from build123d import *

# Parameters (mm, degrees)
SKETCH2_W               = 15.875
SKETCH2_H               = 79.375
SKETCH2_R               = 1.7272
SKETCH2_W_2             = 25.4
SKETCH2_H_2             = 6.35
BOSS_EXTRUDE1_DEPTH     = 69.85
SKETCH3_W               = 19.05
SKETCH3_H               = 12.7
CUT_EXTRUDE1_DEPTH      = 127
SKETCH4_R               = 2.2950679
CUT_EXTRUDE2_DEPTH      = 127
CHAMFER1_SIZE           = 6.35
FILLET2_R               = 6.35
CUT_EXTRUDE3_DEPTH      = 6.35
CUT_EXTRUDE3_DEPTH_BACK = 6.35
SKETCH8_R               = 2.4
SKETCH10_W              = 9.525
SKETCH10_H              = 4.699
BOSS_EXTRUDE2_DEPTH     = 12.7
SKETCH12_R              = 0.8763
CUT_EXTRUDE4_DEPTH      = 132.769283049
CHAMFER2_SIZE           = 4.7752
CHAMFER2_SIZE_2         = 12.7
CHAMFER3_SIZE           = 4.70154
CHAMFER4_SIZE           = 6.35
CHAMFER4_SIZE_2         = 12.7
CUT_EXTRUDE5_DEPTH      = 0.254
CUT_EXTRUDE6_DEPTH      = 0.254


# Some blends are built 0.0001 mm under size
with BuildPart() as part:
    # Sketch2 → Boss-Extrude1 (new body)
    # profile 1 of 2: a face of its own
    with BuildSketch(Plane.ZY.offset(62.053242547)):
        with Locations((17.149745439, 79.910239505)):
            Rectangle(SKETCH2_W, SKETCH2_H)
        with Locations((17.149745439, 113.247739505)):
            Circle(SKETCH2_R, mode=Mode.SUBTRACT)
        with Locations((17.149745439, 71.972739505)):
            Circle(SKETCH2_R, mode=Mode.SUBTRACT)
    # profile 2 of 2: a face of its own
    with BuildSketch(Plane.ZY.offset(62.053242547)):
        with Locations((-3.487754561, 68.797739505)):
            Rectangle(SKETCH2_W_2, SKETCH2_H_2)
    extrude(amount=-BOSS_EXTRUDE1_DEPTH)

    # Sketch3 → Cut-Extrude1 (cut)
    with BuildSketch(Plane(origin=(0, 0, 9.212245439), x_dir=(-1, 0, 0), z_dir=(0, 0, -1))):
        with Locations((27.128242547, 52.922739505)):
            Rectangle(SKETCH3_W, SKETCH3_H)
    extrude(amount=-CUT_EXTRUDE1_DEPTH, mode=Mode.SUBTRACT)

    # Sketch4 → Cut-Extrude2 (cut)
    with BuildSketch(Plane(origin=(7.796757453, 0, 0), x_dir=(0, 0, -1), z_dir=(1, 0, 0))):
        with Locations(Location((-17.149745439, 52.922739505, 0), (0, 0, 180))):
            Circle(SKETCH4_R)
    extrude(amount=-CUT_EXTRUDE2_DEPTH, mode=Mode.SUBTRACT)

    # Chamfer1
    chamfer1_edges = [part.edges().sort_by_distance(p)[0] for p in [
        (-27.128242547, 59.272739505, 25.087245439),
        (-27.128242547, 46.572739505, 9.212245439),
    ]]
    chamfer(chamfer1_edges, length=CHAMFER1_SIZE - 0.0001)  # a hair under: the kernel refuses the full size

    # Fillet2
    fillet2_edges = [part.edges().sort_by_distance(p)[0] for p in [
        (-27.128242547, 59.272739505, 18.737345439),
        (-27.128242547, 46.572739505, 15.562145439),
    ]]
    fillet(fillet2_edges, radius=FILLET2_R)

    # Sketch8 → Cut-Extrude3 (cut, two sides: drawn at the far end of the back side and taken through both)
    # profile 1 of 5: a face of its own
    with BuildSketch(Plane(origin=(-27.128242547, 59.272739505, 33.482952844), x_dir=(0, 0, 1), z_dir=(-1, 0, 0)).offset(-CUT_EXTRUDE3_DEPTH_BACK)):
        with BuildLine():
            Line((-7.077924175, -7.789561181), (-20.085542155, 7.712314277))
            ThreePointArc((-20.085542155, 7.712314277), (-21.190808514, 7.041102183), (-22.339064084, 6.446418612))
            Line((-22.339064084, 6.446418612), (-9.023677061, -9.422241709))
            Line((-9.023677061, -9.422241709), (-7.077924175, -7.789561181))
        make_face()
    # profile 2 of 5: a face of its own
    with BuildSketch(Plane(origin=(-27.128242547, 59.272739505, 33.482952844), x_dir=(0, 0, 1), z_dir=(-1, 0, 0)).offset(-CUT_EXTRUDE3_DEPTH_BACK)):
        with BuildLine():
            Line((-20.085542155, 7.712314277), (-24.270707405, 12.7))
            Line((-24.270707405, 12.7), (-26.21646029, 11.067319471))
            Line((-26.21646029, 11.067319471), (-22.339064084, 6.446418612))
            ThreePointArc((-22.339064084, 6.446418612), (-21.190808514, 7.041102183), (-20.085542155, 7.712314277))
        make_face()
    # profile 3 of 5: a face of its own
    with BuildSketch(Plane(origin=(-27.128242547, 59.272739505, 33.482952844), x_dir=(0, 0, 1), z_dir=(-1, 0, 0)).offset(-CUT_EXTRUDE3_DEPTH_BACK)):
        Polygon((-26.21646029, 11.067319471), (-24.270707405, 12.7), (-27.58644192, 12.7), align=None)
    # profile 4 of 5: a face of its own
    with BuildSketch(Plane(origin=(-27.128242547, 59.272739505, 33.482952844), x_dir=(0, 0, 1), z_dir=(-1, 0, 0)).offset(-CUT_EXTRUDE3_DEPTH_BACK)):
        with BuildLine():
            ThreePointArc((-11.470707405, 23.65), (-13.762240918, 14.591506693), (-20.085542155, 7.712314277))
            Line((-20.085542155, 7.712314277), (-7.077924175, -7.789561181))
            Line((-7.077924175, -7.789561181), (9.239394359, 5.902294783))
            Line((9.239394359, 5.902294783), (-15.927560764, 35.895103965))
            ThreePointArc((-15.927560764, 35.895103965), (-12.619562979, 30.16548373), (-11.470707405, 23.65))
        make_face()
    # profile 5 of 5: a face of its own
    with BuildSketch(Plane(origin=(-27.128242547, 59.272739505, 33.482952844), x_dir=(0, 0, 1), z_dir=(-1, 0, 0)).offset(-CUT_EXTRUDE3_DEPTH_BACK)):
        with BuildLine():
            Line((-27.58644192, 12.7), (-24.270707405, 12.7))
            Line((-24.270707405, 12.7), (-20.085542155, 7.712314277))
            ThreePointArc((-20.085542155, 7.712314277), (-13.762240918, 14.591506693), (-11.470707405, 23.65))
            ThreePointArc((-11.470707405, 23.65), (-12.619562979, 30.16548373), (-15.927560764, 35.895103965))
            ThreePointArc((-15.927560764, 35.895103965), (-42.128931765, 38.754688915), (-46.109164673, 12.7))
            Line((-46.109164673, 12.7), (-27.58644192, 12.7))
        make_face()
        with Locations((-30.520707405, 23.65)):
            Circle(SKETCH8_R, mode=Mode.SUBTRACT)
    extrude(amount=CUT_EXTRUDE3_DEPTH + CUT_EXTRUDE3_DEPTH_BACK, mode=Mode.SUBTRACT)

    # Sketch10 → Boss-Extrude2 (add)
    with BuildSketch(Plane(origin=(0, 0, 9.212245439), x_dir=(-1, 0, 0), z_dir=(0, 0, -1))):
        with Locations((46.262342601, 74.322239505)):
            Rectangle(SKETCH10_W, SKETCH10_H)
        with Locations((46.262342601, 102.311439505)):
            Rectangle(SKETCH10_W, SKETCH10_H)
    extrude(amount=BOSS_EXTRUDE2_DEPTH)

    # Sketch12 → Cut-Extrude4 (cut, through all)
    with BuildSketch(Plane(origin=(-41.499842601, 0, 0), x_dir=(0, 0, -1), z_dir=(1, 0, 0))):
        with Locations((-2.862245439, 101.816839505)):
            Circle(SKETCH12_R)
        with Locations((-2.862245439, 74.816839505)):
            Circle(SKETCH12_R)
    extrude(amount=-CUT_EXTRUDE4_DEPTH, mode=Mode.SUBTRACT)

    # Chamfer2
    # the kernel refuses this chamfer: 12.7, 4.7752 mm, written as the material it adds along each edge
    with BuildSketch(Plane(origin=(-41.499842601, 104.660939505, 9.212245439), x_dir=(0, 0.9954252149618871, 0.09554392402492679), z_dir=(-1, 0, 0))) as chamfer2_piece_1:
        Polygon((CHAMFER2_SIZE * 0.995425214962, CHAMFER2_SIZE * 0.0955439240249), (-CHAMFER2_SIZE_2 * 0.0955439240249, CHAMFER2_SIZE_2 * 0.995425214962), (0, 0), align=None)
    extrude(amount=9.525)

    # Chamfer3
    # the kernel refuses this chamfer: 4.70154 mm, written as the material it adds along each edge
    with BuildSketch(Plane(origin=(-62.053242547, 71.972739505, 9.212245439), x_dir=(0, 0.9996219169112968, 0.02749587661058452), z_dir=(1, 0, 0))) as chamfer3_piece_1_section:
        Polygon((CHAMFER3_SIZE * 0.999621916911, -CHAMFER3_SIZE * 0.0274958766106), (-CHAMFER3_SIZE * 0.0274958766106, -CHAMFER3_SIZE * 0.999621916911), (0, 0), align=None)
    chamfer3_piece_1 = extrude(amount=23.119270381, mode=Mode.PRIVATE)
    chamfer3_piece_1 = split(chamfer3_piece_1, bisect_by=Plane(origin=(-41.499842601, 76.672586172, 9.211398772), z_dir=(-1, 0, 0)), keep=Keep.TOP, mode=Mode.PRIVATE)
    add(chamfer3_piece_1)
    with BuildSketch(Plane(origin=(-20.778242547, 71.972739505, 9.212245439), x_dir=(0, 0.9996219169112968, 0.02749587661058452), z_dir=(1, 0, 0))) as chamfer3_piece_2:
        Polygon((CHAMFER3_SIZE * 0.999621916911, -CHAMFER3_SIZE * 0.0274958766106), (-CHAMFER3_SIZE * 0.0274958766106, -CHAMFER3_SIZE * 0.999621916911), (0, 0), align=None)
    extrude(amount=28.575)

    # Chamfer4
    # the kernel refuses this chamfer: 12.7, 6.35 mm, written as the material it adds along each edge
    with BuildSketch(Plane(origin=(-51.024842601, 142.326966202, 9.212245439), x_dir=(-0.9976223042390326, -2.633779610739709e-14, 0.06891834360170875), z_dir=(0, -1, 0))) as chamfer4_piece_1_section:
        Polygon((CHAMFER4_SIZE * 0.997622304239, CHAMFER4_SIZE * 0.0689183436017), (-CHAMFER4_SIZE_2 * 0.0689183436017, CHAMFER4_SIZE_2 * 0.997622304239), (0, 0), align=None)
    chamfer4_piece_1 = extrude(amount=42.365026697, mode=Mode.PRIVATE)
    chamfer4_piece_1 = split(chamfer4_piece_1, bisect_by=Plane(origin=(-53.26388473, 107.534062678, 4.153530473), z_dir=(0, -0.9360210850035494, 0.35194392796122825)), keep=Keep.TOP, mode=Mode.PRIVATE)
    chamfer4_piece_1 = chamfer4_piece_1 - Plane(origin=(-53.26388473, 101.816839505, 2.862245439), x_dir=(0, 0, -1), z_dir=(1, 0, 0)) * Cylinder(0.8763, 136, mode=Mode.PRIVATE)
    add(chamfer4_piece_1)

    # Sketch13 → Cut-Extrude5 (cut)
    with BuildSketch(Plane(origin=(7.796757453, 0, 0), x_dir=(0, 0, -1), z_dir=(1, 0, 0))):
        Polygon((16.187754561, 65.622739505), (16.187754561, 71.972739505), (-4.510705439, 71.972739505), (-9.212245439, 76.674279505), (-9.212245439, 119.597739505), (-25.087245439, 119.597739505), (-25.087245439, 40.222739505), (-9.212245439, 40.222739505), (-9.212245439, 65.622739505), align=None)
    extrude(amount=-CUT_EXTRUDE5_DEPTH, mode=Mode.SUBTRACT)

    # Sketch14 → Cut-Extrude6 (cut)
    with BuildSketch(Plane.ZY.offset(62.053242547)):
        Polygon((-16.187754561, 71.972739505), (-16.187754561, 65.622739505), (9.212245439, 65.622739505), (9.212245439, 40.222739505), (25.087245439, 40.222739505), (25.087245439, 119.597739505), (9.212245439, 119.597739505), (9.212245439, 76.674279505), (4.510705439, 71.972739505), align=None)
    extrude(amount=-CUT_EXTRUDE6_DEPTH, mode=Mode.SUBTRACT)


solid = part.part
Can you work these out from the model? Positions are in its coordinate system, mm. A direction names the side the tool comes from. Round coordinates to 2 decimals unless told otherwise and drop trailing zeros. Loops run counter-clockwise (first coordinate to the right, second up) from the corner with the lowest first, then second, coordinate; pieces in that order, holes last. Notation, with made-up numbers: (-17, 61.5) - (27, 61.5) arc R11 cw to (27, 71.5) - close; hole circle Ø1 at (25, 64). An arc over 180 degrees is marked (long way). Write item = value, one per line. Start each with the question number.
(1) If I drill on probe 1 along X at (y, z) = (58, 16.5); probe 2 along X at (y, z) = (87, 17); probe 3 along Y at (x, z) = (-22.5, 10), over which ranges is the centre line in solid material (lowest first)? Write a range as [from, to].
(2) If we section it at C-C (y = 92.5): Please give me the cut outline in (x, z), and give its area (3 significant figures).
(3) For faces 1 (the face through (-27, 59.273, 13)), 2 (the face through (-19.213, 63.409, 22.874)), 3 (the face through (-46, 76.672, 3)), 4 (the face through (-41.5, 103, 3)), which set-ups out of +Z, -Z, +X, -X, +Y, -Y let a thin tool reach every point of the face, with its end or its side?
(4) For P1, Ø2, axis at y = 71.97, z = 17.15, coming from the +X side; P2, Ø1.4, axis at x = -47, y = 102.5, coming from the -Z side; P3, Ø3, axis at x = -44.5, z = 0, coming from the +Y side; P4, Ø1.4, axis at y = 74, z = 1, coming from the -X side, each with a flat end and sliding along its axis, tell me the tip position at first contact or that it passes through.
(5) If we mould it in two halves opening along Y, with no side actions, what happens to faces 5 (the face through (-28, 61, 9.212)), 6 (the face through (-17.603, 56, 17)), 7 (the face through (-47.6, 107.1, 3))? For each: released by +Y, released by -Y, zero draft, split by the parting line, or undercut.
(6) If we section it at D-D (y = 67.5): Please give me the cut outline in (x, z).
(7) If we section it at A-A (x = -32): Give the number of separate pieces and of enclosed holes in the cut face, and give its area (3 significant figures).
Ans:
q1.probe_1 = [-61.8, -36.65], [-17.6, 7.54]
q1.probe_2 = [-61.8, -33.48], [-20.78, 7.54]
q1.probe_3 = [40.22, 41.01], [59.27, 67.08], [100.63, 119.6]
q2.outline = (-61.8, 9.21) - (-33.48, 9.21) - (-33.48, 19.79) - (-20.78, 19.79) - (-20.78, 9.21) - (7.54, 9.21) - (7.54, 25.09) - (-61.8, 25.09) - close
q2.area = 966 mm²
q3.face_1 = +Z, -Z
q3.face_2 = +Z
q3.face_3 = -Z, +X, -X
q3.face_4 = -Z, +X, +Y
q4.P1 = through
q4.P2 = -3.49
q4.P3 = 106.54
q4.P4 = -51.02
q5.face_5 = zero draft
q5.face_6 = undercut
q5.face_7 = released by +Y
q6.outline = (-61.8, -16.19) - (7.54, -16.19) - (7.54, 25.09) - (-20.78, 25.09) - (-20.78, 9.65) - (-33.48, 9.65) - (-33.48, 25.09) - (-61.8, 25.09) - close
q7.separate_pieces = 3
q7.enclosed_holes = 1
q7.area = 650 mm²
